from build123d import *

# Parameters (mm, degrees)
CROQUIS1_W              = 15
CROQUIS1_H              = 15
SALIENTE_EXTRUIR1_DEPTH = 55
CORTAR_EXTRUIR1_DEPTH   = 58.5
CROQUIS3_R              = 2.5
CORTAR_EXTRUIR2_DEPTH   = 58.5
CORTAR_EXTRUIR3_DEPTH   = 58.5


with BuildPart() as part:
    # Croquis1 → Saliente-Extruir1 (new, symmetric)
    with BuildSketch(Plane(origin=(0, 0, 0), x_dir=(0, 0, -1), z_dir=(1, 0, 0))):
        Rectangle(CROQUIS1_W, CROQUIS1_H)
    extrude(amount=SALIENTE_EXTRUIR1_DEPTH, both=True)

    # Croquis2 → Cortar-Extruir1 (cut, through all)
    with BuildSketch(Plane.XY.offset(7.5)):
        with BuildLine():
            ThreePointArc((-43.802977877, -1.239902926), (-40, -4), (-36.197022123, -1.239902926))
            Line((-36.197022123, -1.239902926), (-43.802977877, -1.239902926))
        make_face()
        with BuildLine():
            Line((-43.802977877, -1.239902926), (-36.197022123, -1.239902926))
            ThreePointArc((-36.197022123, -1.239902926), (-36.049562587, -0.627729437), (-36, 0))
            ThreePointArc((-36, 0), (-36.049562587, 0.627729437), (-36.197022123, 1.239902926))
            Line((-36.197022123, 1.239902926), (-43.802977877, 1.239902926))
            ThreePointArc((-43.802977877, 1.239902926), (-44, 0), (-43.802977877, -1.239902926))
        make_face()
        with BuildLine():
            Line((-43.802977877, 1.239902926), (-36.197022123, 1.239902926))
            ThreePointArc((-36.197022123, 1.239902926), (-40, 4), (-43.802977877, 1.239902926))
        make_face()
        with BuildLine():
            Line((-36.197022123, -1.239902926), (-25, -1.239902926))
            Line((-25, -1.239902926), (-25, 1.239902926))
            Line((-25, 1.239902926), (-36.197022123, 1.239902926))
            ThreePointArc((-36.197022123, 1.239902926), (-36.049562587, 0.627729437), (-36, 0))
            ThreePointArc((-36, 0), (-36.049562587, -0.627729437), (-36.197022123, -1.239902926))
        make_face()
        with BuildLine():
            Line((-55, -1.239902926), (-43.802977877, -1.239902926))
            ThreePointArc((-43.802977877, -1.239902926), (-44, 0), (-43.802977877, 1.239902926))
            Line((-43.802977877, 1.239902926), (-55, 1.239902926))
            Line((-55, 1.239902926), (-55, -1.239902926))
        make_face()
    extrude(amount=-CORTAR_EXTRUIR1_DEPTH, mode=Mode.SUBTRACT)

    # Croquis3 → Cortar-Extruir2 (cut, through all)
    with BuildSketch(Plane(origin=(0, 7.5, 0), x_dir=(1, 0, 0), z_dir=(0, 1, 0))):
        with Locations(Location((-48.75, 0, 0), (0, 0, 270))):
            Circle(CROQUIS3_R)
    extrude(amount=-CORTAR_EXTRUIR2_DEPTH, mode=Mode.SUBTRACT)

    # Croquis4 → Cortar-Extruir3 (cut, through all)
    with BuildSketch(Plane.XY.offset(7.5)):
        with BuildLine():
            Line((37, 3.175), (43, 3.175))
            ThreePointArc((43, 3.175), (46.175, 0), (43, -3.175))
            Line((43, -3.175), (37, -3.175))
            ThreePointArc((37, -3.175), (33.825, 0), (37, 3.175))
        make_face()
    extrude(amount=-CORTAR_EXTRUIR3_DEPTH, mode=Mode.SUBTRACT)


solid = part.part
Work out the finished part from the listing and answer in its coordinate system (mm). A direction names the side the tool comes from. Give positions to 0.01 mm unless a question says otherwise; leave off trailing zeros. Order: outer loops, then holes, each group sorted by start corner. A loop starts at its lowest first (then second) coordinate and runs counter-clockwise, first axis right, second up. Notation, with made-up numbers: M -29,82.5 L 1,82.5 A14 ccw 1,95.5 Z; hole C 67,79 d4. An arc over 180 degrees is marked long. Return JSON: item names as keys, results as strings.
Q1. Find section B-B, the plane y = 0. Write down the section's boundary in (x, z) (3 decimals).
Answer below:
{"outline": "M -25,-7.5 L 33.825,-7.5 L 33.825,7.5 L -25,7.5 Z; M 46.175,-7.5 L 55,-7.5 L 55,7.5 L 46.175,7.5 Z"}
Q2. Find section C-C, the plane x = -48.75. Write down the section's boundary in (y, z).
Answer below:
{"outline": "M -7.5,-7.5 L -1.24,-7.5 L -1.24,-2.5 L -7.5,-2.5 Z; M -7.5,2.5 L -1.24,2.5 L -1.24,7.5 L -7.5,7.5 Z; M 1.24,-7.5 L 7.5,-7.5 L 7.5,-2.5 L 1.24,-2.5 Z; M 1.24,2.5 L 7.5,2.5 L 7.5,7.5 L 1.24,7.5 Z"}
Q3. The mould has two halves that part along Z. Classify faces 1 (the face through (-51.2, -4.3, -0.5)), 2 (the face through (-55, 4, 0)), 3 (the face through (1, 0, 7.5)): pulls with the +Z half, pulls with the -Z half, needs draft (parallel to the pull), parting line crosses it, or undercut.
Answer below:
{"face 1": "undercut", "face 2": "needs draft", "face 3": "pulls with the +Z half"}
Q4. Find the intervals of material crossed by line 1 along Y through (x, z) = (-26, 5); line 2 along X through (y, z) = (2, -0.25); line 3 along X through (y, z) = (-2, -3), in increasing order. Write a range as [from, to].
Answer below:
{"line 1": "y = [-7.5, -1.24], [1.24, 7.5]", "line 2": "x = [-55, -51.24], [-46.26, -43.46], [-36.54, 34.53], [45.47, 55]", "line 3": "x = [-55, -43.46], [-36.54, 34.53], [45.47, 55]"}
Q5. This flat-tipped pin is pushed along its axis until it touches: pin 1 (0.7 mm diameter, centred on y = 0.5, z = 0, fed in from -X). Where does it stop, or does it pass through?
Answer below:
{"pin 1": "stops at x = -25"}
Q6. Find section D-D, the plane x = 45. Write down the section's boundary in (y, z), and give its area (3 significant figures).
Answer below:
{"outline": "M -7.5,-7.5 L -2.47,-7.5 L -2.47,7.5 L -7.5,7.5 Z; M 2.47,-7.5 L 7.5,-7.5 L 7.5,7.5 L 2.47,7.5 Z", "area": "151 mm^2"}
Q7. Which of the six approach directions +Z, -Z, +X, -X, +Y, -Y give full straight-line access (tool end or side, diameter ignored) to faces 4 (the face through (-40, -4, 0)), 5 (the face through (-55, -4, 0)), 6 (the face through (-31, -1.24, 0))?
Answer below:
{"face 4": "+Z, -Z", "face 5": "+Z, -Z, -X, +Y, -Y", "face 6": "+Z, -Z, -X"}
Q8. Find section A-A, the plane z = -1.5. Write down the section's boundary in (x, y) (3 decimals).
Answer below:
{"outline": "M -55,-7.5 L -50.75,-7.5 L -50.75,-1.24 L -55,-1.24 Z; M -55,1.24 L -50.75,1.24 L -50.75,7.5 L -55,7.5 Z; M -46.75,-7.5 L 55,-7.5 L 55,7.5 L -46.75,7.5 L -46.75,1.24 L -43.803,1.24 A4 cw -36.197,1.24 L -25,1.24 L -25,-1.24 L -36.197,-1.24 A4 cw -43.803,-1.24 L -46.75,-1.24 Z; hole M 37,-3.175 L 43,-3.175 A3.175 ccw 43,3.175 L 37,3.175 A3.175 ccw Z"}
